```python
from build123d import *

# Parameters (mm, degrees)
PAD_DEPTH = 10
FILLET_R  = 0.5


with BuildPart() as part:
    # Sketch → Pad (new body)
    with BuildSketch(Plane.XY):
        Polygon((-7.5, 23.28312), (-7.5, 16.28312), (-1.5, 16.28312), (-1.5, 14.93312), (-2.7, 14.93312), (-2.7, 12.63312), (-1.5, 12.63312), (-1.5, 11.28312), (1.5, 11.28312), (1.5, 12.63312), (2.7, 12.63312), (2.7, 14.93312), (1.5, 14.93312), (1.5, 16.28312), (7.5, 16.28312), (7.5, 23.28312), (5.5, 23.28312), (5.5, 19.28312), (-5.5, 19.28312), (-5.5, 23.28312), align=None)
    extrude(amount=PAD_DEPTH)

    # Fillet
    fillet_edges = [part.edges().sort_by_distance(p)[0] for p in [
        (2.7, 12.63312, 5),
        (2.7, 14.93312, 5),
        (2.7, 13.78312, 0),
        (2.7, 13.78312, 10),
        (1.5, 11.28312, 5),
        (-1.5, 11.28312, 5),
        (0, 11.28312, 0),
        (0, 11.28312, 10),
        (-2.7, 13.78312, 0),
        (1.5, 12.63312, 5),
        (1.5, 14.93312, 5),
        (-1.5, 12.63312, 5),
        (-1.5, 14.93312, 5),
        (-2.7, 14.93312, 5),
        (-2.7, 12.63312, 5),
        (1.5, 16.28312, 5),
        (7.5, 16.28312, 5),
        (-1.5, 16.28312, 5),
        (-7.5, 16.28312, 5),
        (-7.5, 23.28312, 5),
        (7.5, 23.28312, 5),
        (5.5, 23.28312, 5),
        (-5.5, 23.28312, 5),
        (6.5, 23.28312, 0),
        (7.5, 19.78312, 0),
        (-6.5, 23.28312, 0),
        (-7.5, 19.78312, 0),
        (-7.5, 19.78312, 10),
        (-6.5, 23.28312, 10),
        (6.5, 23.28312, 10),
        (7.5, 19.78312, 10),
        (-4.5, 16.28312, 10),
        (4.5, 16.28312, 10),
        (-2.7, 13.78312, 10),
        (0, 19.28312, 10),
        (0, 19.28312, 0),
        (-5.5, 21.28312, 0),
        (5.5, 21.28312, 0),
        (5.5, 21.28312, 10),
        (-5.5, 21.28312, 10),
    ]]
    fillet(fillet_edges, radius=FILLET_R)


solid = part.part
```
Geometry: final body of the model. Coordinates: model frame, mm. A direction names the side the tool comes from. Round coordinates to 2 decimals unless told otherwise and drop trailing zeros. Loops run counter-clockwise (first coordinate to the right, second up) from the corner with the lowest first, then second, coordinate; pieces in that order, holes last.
Item 1: Mould query, pull axis X, two halves, no side actions, for faces 1 (the flat face through (-5.5, 21, 5)), 2 (the flat face through (-5, 16.283, 5)), 3 (the flat face through (2.7, 14, 5)). Classes: released by +X, released by -X, zero draft, split by the parting line, or undercut.
Checked values:
face 1: undercut
face 2: zero draft
face 3: released by +X
Item 2: Line query: L1, parallel to X at y = 22, z = 7.5; L2, parallel to Y at x = 3.25, z = 6.75; L3, parallel to Y at x = -2, z = 3. Output: solid intervals per line, ascending.
Checked values:
L1: x = -7.5 to -5.5, 5.5 to 7.5
L2: y = 16.28 to 19.28
L3: y = 12.63 to 14.93, 16.28 to 19.28
Item 3: Reachability of faces 4 (the flat face through (0, 19.283, 5)), 5 (the flat face through (-2.7, 14, 5)), 6 (the flat face through (0, 17, 0)) from +Z, -Z, +X, -X, +Y, -Y: full face, straight path, thin tool, end or side. Return the list, or none.
Checked values:
face 4: +Z, -Z, +Y
face 5: +Z, -Z, -X, -Y
face 6: -Z, +X, -X, +Y, -Y
Item 4: Section B-B, the plane x = 0.5. Output: boundary loops of the cut face in (y, z), plus the area to 3 significant figures.
Checked values:
outline: (11.28, 0.5) arc R0.5 ccw to (11.78, 0) - (18.78, 0) arc R0.5 ccw to (19.28, 0.5) - (19.28, 9.5) arc R0.5 ccw to (18.78, 10) - (11.78, 10) arc R0.5 ccw to (11.28, 9.5) - close
area: 79.8 mm2
Item 5: Contact query for flat-ended pins moving along their axis: P1, Ø1.4, axis at y = 14, z = 7, coming from the -X side; P2, Ø1.5, axis at x = -5.5, z = 3.5, coming from the -Y side; P3, Ø3, axis at x = 2.5, z = 7.5, coming from the +Y side; P4, Ø1, axis at x = 1.5, y = 20, coming from the -Z side. Output: stop coordinate, or through.
Checked values:
P1: stops at x = -2.7
P2: stops at y = 16.28
P3: stops at y = 19.28
P4: passes through
Item 6: Section D-D, the plane x = -4.75. Output: boundary loops of the cut face in (y, z), plus the area to 3 significant figures.
Checked values:
outline: (16.28, 0) - (18.78, 0) arc R0.5 ccw to (19.28, 0.5) - (19.28, 9.5) arc R0.5 ccw to (18.78, 10) - (16.78, 10) arc R0.5 ccw to (16.28, 9.5) - close
area: 29.8 mm2
Item 7: Section A-A, the plane y = 20.5. Output: boundary loops of the cut face in (x, z).
Checked values:
outline: (-7.5, 0.5) arc R0.5 ccw to (-7, 0) - (-6, 0) arc R0.5 ccw to (-5.5, 0.5) - (-5.5, 9.5) arc R0.5 ccw to (-6, 10) - (-7, 10) arc R0.5 ccw to (-7.5, 9.5) - close; (5.5, 0.5) arc R0.5 ccw to (6, 0) - (7, 0) arc R0.5 ccw to (7.5, 0.5) - (7.5, 9.5) arc R0.5 ccw to (7, 10) - (6, 10) arc R0.5 ccw to (5.5, 9.5) - close
Item 8: Section C-C, the plane y = 13.5. Output: boundary loops of the cut face in (x, z).
Checked values:
outline: (-2.7, 0.5) arc R0.5 ccw to (-2.2, 0) - (2.2, 0) arc R0.5 ccw to (2.7, 0.5) - (2.7, 9.5) arc R0.5 ccw to (2.2, 10) - (-2.2, 10) arc R0.5 ccw to (-2.7, 9.5) - close
